For this review, use the dimensioned drawing (mm, ordinates from the lowest corner) and the shaded views. Coordinates: 2 decimals unless noted, no trailing zeros. Use one line per item in the form item = value. Start each with the question number.
1. Wall thickness on line 1 (X direction, y = 23.5, z = 0.75) (1 decimal); line 2 (Y direction, x = 16, z = 3); line 3 (Z direction, x = 46.5, y = 7.5) (1 decimal): over which ranges is each line inside the solid? List them lowest first. Write a range as from..to.
2. For pin 1 (1.5 mm diameter, centred on x = 31.5, z = 7, fed in from +Y) (1 decimal); pin 2 (1.5 mm diameter, centred on y = 27.5, z = 6, fed in from -X) (1 decimal); pin 3 (4 mm diameter, centred on x = 20, z = 7.5, fed in from -Y) (1 decimal), all flat-tipped, find the tip position at first contact; note any pin that passes through.
3. The part is to be moulded in two halves that separate along Y. For the marked faces 1 and 2, say which applies: released by +Y, released by -Y, zero draft, split by the parting line, or undercut.
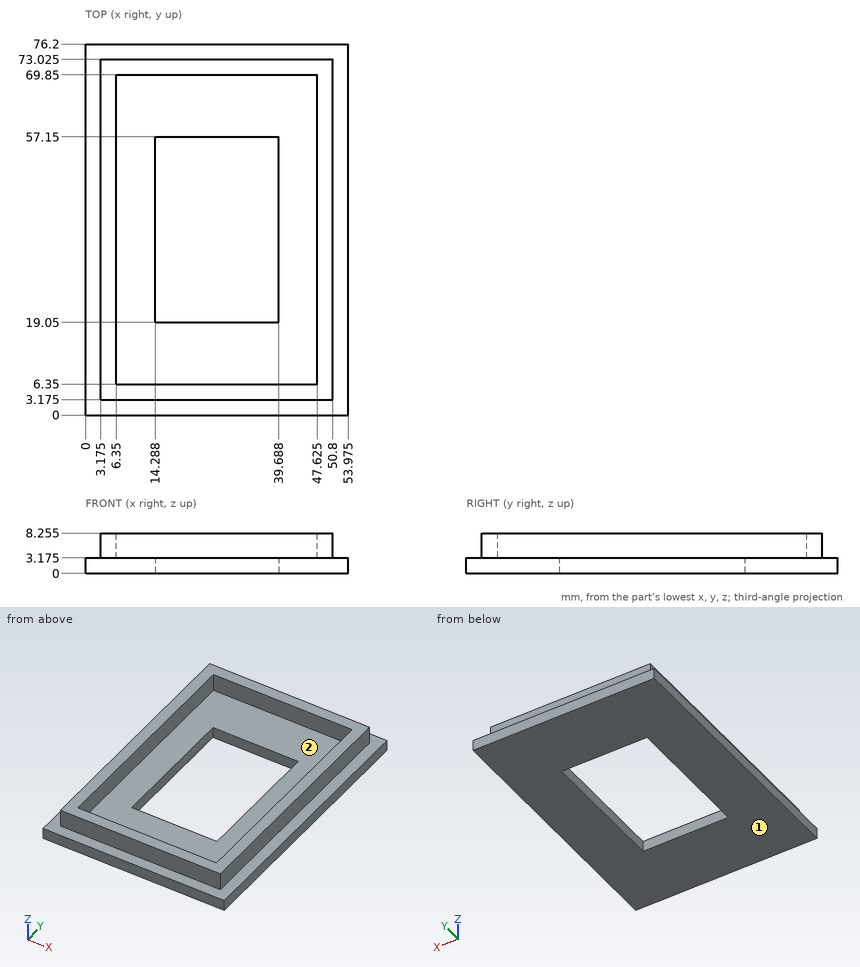
Geometry check:
q1.line_1 = 0..14.3, 39.7..54
q1.line_2 = 0..19.05, 57.15..76.2
q1.line_3 = 0..3.2
q2.pin_1 = 73
q2.pin_2 = 3.2
q2.pin_3 = 3.2
q3.face_1 = zero draft
q3.face_2 = undercut
